Geometry check sheet. Reference: the model listing, model coordinates, mm. A direction names the side the tool comes from. Coordinates: 2 decimals unless noted, no trailing zeros. Loops run counter-clockwise (first coordinate to the right, second up) from the corner with the lowest first, then second, coordinate; pieces in that order, holes last. Notation, with made-up numbers: (-11, 46) - (6, 46) arc R22 ccw to (6, 60) - close; hole circle Ø2 at (72.5, 2.5). An arc over 180 degrees is marked (long way). One line per item, written item: value.
from build123d import *

# Parameters (mm, degrees)
ESBO_O1_R                = 32.5
RESSALTO_EXTRUS_O1_DEPTH = 4
ESBO_O2_W                = 4
ESBO_O2_H                = 8
ESBO_O2_R                = 1
RESSALTO_EXTRUS_O3_DEPTH = 4.5
ESBO_O3_W                = 23
ESBO_O3_H                = 13
CORTE_EXTRUS_O1_DEPTH    = 1
ESBO_O4_W                = 40
ESBO_O4_H                = 6
RESSALTO_EXTRUS_O4_DEPTH = 71
ESBO_O5_R                = 4.5
CORTE_EXTRUS_O2_DEPTH    = 61
CORTE_EXTRUS_O3_DEPTH    = 3
FILETE1_R                = 5


with BuildPart() as part:
    # Esboço1 → Ressalto-extrusão1 (new body)
    with BuildSketch(Plane.XY):
        Circle(ESBO_O1_R)
        with BuildLine():
            ThreePointArc((5.921389022, 2.680886429), (-6.5, 0), (5.921389022, -2.680886429))
            ThreePointArc((5.921389022, -2.680886429), (9.242616034, 0), (5.921389022, 2.680886429))
        make_face(mode=Mode.SUBTRACT)
    extrude(amount=RESSALTO_EXTRUS_O1_DEPTH)

    # Esboço2 → Ressalto-extrusão3 (add)
    with BuildSketch(Plane.XY.offset(4)):
        with Locations((-8.5, 0)):
            Rectangle(ESBO_O2_W, ESBO_O2_H)
        with Locations((-8.5, 0)):
            Circle(ESBO_O2_R, mode=Mode.SUBTRACT)
        with Locations((18.5, 0)):
            Rectangle(ESBO_O2_W, ESBO_O2_H)
        with Locations((18.5, 0)):
            Circle(ESBO_O2_R, mode=Mode.SUBTRACT)
    extrude(amount=RESSALTO_EXTRUS_O3_DEPTH)

    # Esboço3 → Corte-extrusão1 (cut)
    with BuildSketch(Plane.XY.offset(4)):
        with Locations((5, 0)):
            Rectangle(ESBO_O3_W, ESBO_O3_H)
    extrude(amount=-CORTE_EXTRUS_O1_DEPTH, mode=Mode.SUBTRACT)

    # Esboço4 → Ressalto-extrusão4 (add)
    with BuildSketch(Plane.XY.offset(4)):
        with Locations((0, -11.5)):
            Rectangle(ESBO_O4_W, ESBO_O4_H)
    extrude(amount=RESSALTO_EXTRUS_O4_DEPTH)

    # Esboço5 → Corte-extrusão2 (cut)
    with BuildSketch(Plane.XZ.offset(14.5)):
        with Locations((0, 56.5)):
            Circle(ESBO_O5_R)
    extrude(amount=-CORTE_EXTRUS_O2_DEPTH, mode=Mode.SUBTRACT)

    # Esboço6 → Corte-extrusão3 (cut)
    with BuildSketch(Plane.XZ.offset(14.5)):
        with BuildLine():
            Line((0, 64.5), (-10.70310615, 70.032504242))
            ThreePointArc((-10.70310615, 70.032504242), (-13.151971512, 69.651971512), (-13.532504242, 67.20310615))
            Line((-13.532504242, 67.20310615), (-8, 56.5))
            Line((-8, 56.5), (-13.532504242, 45.79689385))
            ThreePointArc((-13.532504242, 45.79689385), (-13.151971512, 43.348028488), (-10.70310615, 42.967495758))
            Line((-10.70310615, 42.967495758), (0, 48.5))
            Line((0, 48.5), (10.70310615, 42.967495758))
            ThreePointArc((10.70310615, 42.967495758), (13.151971512, 43.348028488), (13.532504242, 45.79689385))
            Line((13.532504242, 45.79689385), (8, 56.5))
            Line((8, 56.5), (13.532504242, 67.20310615))
            ThreePointArc((13.532504242, 67.20310615), (13.151971512, 69.651971512), (10.70310615, 70.032504242))
            Line((10.70310615, 70.032504242), (0, 64.5))
        make_face()
    extrude(amount=-CORTE_EXTRUS_O3_DEPTH, mode=Mode.SUBTRACT)

    # Filete1
    filete1_edges = [part.edges().sort_by_distance(p)[0] for p in [
        (20, -11.5, 75),
        (-20, -11.5, 75),
    ]]
    fillet(filete1_edges, radius=FILETE1_R)


solid = part.part
(1) Go/stop test with flat-tipped pins: pin 1 Ø1.6 at (y, z) = (-1, 6.5) entering from -X; pin 2 Ø3 at (y, z) = (-12.5, 26) entering from +X; pin 3 Ø12 at (x, y) = (-5, -23.5) entering from +Z. Record where each tip stops, or that it passes through.
Reply:
pin 1: x = -10.5
pin 2: x = 20
pin 3: z = 4
(2) Release check for a two-part mould opening along Y. For faces 1 (the face through (-9, 4, 6)), 2 (the face through (17.6, 0.9, 8.5)), 3 (the face through (12, 0, 3)) record: pulls with the +Y half, pulls with the -Y half, needs draft (parallel to the pull), parting line crosses it, or undercut.
Reply:
face 1: pulls with the +Y half
face 2: needs draft
face 3: undercut
(3) Material ranges on probe 1 along Y at (x, z) = (18.5, 5.8); probe 2 along Z at (x, y) = (-5, -7); probe 3 along Y at (x, z) = (9, 13), recorded low to high. Write a range as from..to.
Reply:
probe 1: -14.5..-8.5, -4..-1, 1..4
probe 2: 0..4
probe 3: -14.5..-8.5
(4) Cross-section at A-A on x = -1. Record the cut outline in (y, z).
Reply:
outline: (-32.48, 0) - (-6.42, 0) - (-6.42, 3) - (-6.5, 3) - (-6.5, 4) - (-8.5, 4) - (-8.5, 52.11) - (-11.5, 52.11) - (-11.5, 47.98) - (-14.5, 47.98) - (-14.5, 4) - (-32.48, 4) - close; (-14.5, 65.02) - (-11.5, 65.02) - (-11.5, 60.89) - (-8.5, 60.89) - (-8.5, 75) - (-14.5, 75) - close; (6.42, 0) - (32.48, 0) - (32.48, 4) - (6.5, 4) - (6.5, 3) - (6.42, 3) - close
(5) Cross-section at C-C on z = 54. Record the cut outline in (x, y).
Reply:
outline: (-20, -14.5) - (-9.29, -14.5) - (-9.29, -11.5) - (-3.74, -11.5) - (-3.74, -8.5) - (-20, -8.5) - close; (3.74, -11.5) - (9.29, -11.5) - (9.29, -14.5) - (20, -14.5) - (20, -8.5) - (3.74, -8.5) - close
(6) Access from +Z, -Z, +X, -X, +Y, -Y to the whole of each face (thin tool, end or side, straight path). Record for faces 4 (the face through (-9, 0, 4)), 5 (the face through (-9, -4, 6)), 6 (the face through (10.805, -13.021, 51.074)), 7 (the face through (-7.6, 0.9, 8.5)).
Reply:
face 4: +Z
face 5: +Z, +X, -X
face 6: -Y
face 7: +Z, +X, -X, +Y
(7) Cross-section at B-B on y = -5.5. Record the cut outline in (x, z), and give its area (3 significant figures).
Reply:
outline: (-32.03, 0) - (-3.46, 0) - (-3.46, 3) - (-6.5, 3) - (-6.5, 4) - (-32.03, 4) - close; (3.46, 0) - (32.03, 0) - (32.03, 4) - (16.5, 4) - (16.5, 3) - (3.46, 3) - close
area: 212 mm2
(8) Cross-section at D-D on z = 15. Record the cut outline in (x, y).
Reply:
outline: (-20, -14.5) - (20, -14.5) - (20, -8.5) - (-20, -8.5) - close
